```python
from build123d import *

# Parameters (mm, degrees)
SKETCH1_R         = 3.175
EXTRUDE1_DEPTH    = 7.14375
EXTRUDE2_DEPTH    = 2.286
CIRPATTERN1_COUNT = 3


with BuildPart() as part:
    # Sketch1 → Extrude1 (new body)
    with BuildSketch(Plane.XY):
        Polygon((5.657191877, 3.026339728), (0.207708854, 6.412441744), (-5.449483023, 3.386102016), (-5.657191877, -3.026339728), (-0.207708854, -6.412441744), (5.449483023, -3.386102016), align=None)
        Circle(SKETCH1_R, mode=Mode.SUBTRACT)
    extrude(amount=EXTRUDE1_DEPTH)

    # Sketch2 → Extrude2 (cut)
    with BuildSketch(Plane.XY.offset(7.14375)):
        Polygon((-4.410852186, -4.735268522), (2.291891507, 6.051910302), (4.410852186, 4.735268522), (-2.291891507, -6.051910302), align=None)
    extrude2 = extrude(amount=-EXTRUDE2_DEPTH, mode=Mode.SUBTRACT)

    # CirPattern1: Extrude2 ×3 about axis
    cirpattern1_axis = Axis((0, 0, 0), (0, 0, 1))
    for i in range(1, CIRPATTERN1_COUNT):
        add(extrude2.rotate(cirpattern1_axis, i * 360 / CIRPATTERN1_COUNT), mode=Mode.SUBTRACT)


solid = part.part
```
The listing builds one solid part. Answer for the finished solid, in the listing's coordinates (mm). A direction names the side the tool comes from. Round coordinates to 2 decimals unless told otherwise and drop trailing zeros. Write each loop counter-clockwise with the first axis right and the second up, starting at its lowest first coordinate (ties: lowest second). Pieces come first, ordered by that corner, then holes. Notation, with made-up numbers: (86.25, 44) -> (101.25, 44) arc R28 ccw to (101.25, 64) -> close; hole circle Ø4 at (-32, 49). An arc over 180 degrees is marked (long way). Answer as a JSON object with one key per item and string values. Group by question number.
Q1. Straight lines are drawn through the part: line 1 along X through (y, z) = (0, 2.75) (3 decimals); line 2 along Y through (x, z) = (-1.75, 1); line 3 along Y through (x, z) = (0, 3.75) (3 decimals). For each, find the intervals that lie inside material, in ascending order.
Q2. Section B-B (y = 0) is taken. Write down the section's boundary in (x, z) (3 decimals).
Q3. Section C-C (z = 1) is taken. Write down the section's boundary in (x, y) (3 decimals), plus the area to 3 significant figures.
Q4. Which of the six approach directions +Z, -Z, +X, -X, +Y, -Y give full straight-line access (tool end or side, diameter ignored) to faces 1 (the face through (3.31, 2.96, 6.02)), 2 (the face through (-2.58, 4.92, 3.52)), 3 (the face through (2, 4, 4.858))?
Q5. Section A-A (z = 6.75) is taken. Count the separate pieces of the cut face and the enclosed holes in it, plus the area to 3 significant figures.
Q6. Each of these flat-tipped pins is pushed along its axis until it touches: pin 1 Ø3 at (x, y) = (0, -5) entering from -Z; pin 2 Ø3 at (y, z) = (1, 1.5) entering from -X; pin 3 Ø1 at (x, z) = (-4.5, 2.5) entering from +Y; pin 4 Ø2 at (x, y) = (-4.5, 0) entering from +Z. Where does it stop, or does it pass through?
Q7. Section D-D (x = 0) is taken. Write down the section's boundary in (y, z) (3 decimals), plus the area to 3 significant figures.
Q8. Determine the mould class of faces 4 (the face through (3.09, -3.13, 6.02)), 5 (the face through (0, 5, 7.144)), 6 (the face through (-3.31, -2.96, 6.02)), 7 (the face through (-2.971, -4.696, 3.522)) for opening direction X: pulls with the +X half, pulls with the -X half, needs draft (parallel to the pull), parting line crosses it, or undercut.
Check values:
{
 "1": {"line 1": "-5.559 to -3.175, 3.175 to 5.559", "line 2": "-5.45 to -2.65, 2.65 to 5.37", "line 3": "-6.301 to -3.175, 3.175 to 6.301"},
 "2": {"outline": "(-5.559, 0) -> (-3.175, 0) -> (-3.175, 4.858) -> (-5.559, 4.858) -> close; (3.175, 0) -> (5.559, 0) -> (5.559, 4.858) -> (3.175, 4.858) -> close"},
 "3": {"outline": "(-5.657, -3.026) -> (-0.208, -6.412) -> (5.449, -3.386) -> (5.657, 3.026) -> (0.208, 6.412) -> (-5.449, 3.386) -> close; hole circle Ø6.35 at (0, 0)", "area": "75.3 mm^2"},
 "4": {"face 1": "+Z, +Y", "face 2": "+Z, -Z, -X, +Y", "face 3": "+Z"},
 "5": {"separate pieces": "6", "enclosed holes": "0", "area": "38.4 mm^2"},
 "6": {"pin 1": "z = 0", "pin 2": "x = -5.58", "pin 3": "y = 4.16", "pin 4": "z = 4.86"},
 "7": {"outline": "(-6.301, 0) -> (-3.175, 0) -> (-3.175, 7.144) -> (-6.301, 7.144) -> close; (3.175, 0) -> (6.301, 0) -> (6.301, 7.144) -> (3.175, 7.144) -> close", "area": "44.7 mm^2"},
 "8": {"face 4": "undercut", "face 5": "needs draft", "face 6": "undercut", "face 7": "pulls with the -X half"}
}
